Geometry: final body of the model. Coordinates: model frame, mm. Face numbers are marked on the shaded views. Give positions to 0.01 mm unless a question says otherwise; leave off trailing zeros. Order: outer loops, then holes, each group sorted by start corner. A loop starts at its lowest first (then second) coordinate and runs counter-clockwise, first axis right, second up. Notation, with made-up numbers: (-23, 7) - (-11, 7) arc R29 cw to (-11, 32) - close; hole circle Ø1 at (10.25, 7). An arc over 180 degrees is marked (long way). Use one line per item in the form item = value.
from build123d import *

# Parameters (mm, degrees)
BOSS_EXTRUDE2_DEPTH = 2.5
BOSS_EXTRUDE3_DEPTH = 5
BOSS_EXTRUDE4_START = 5
BOSS_EXTRUDE4_DEPTH = 5
SKETCH4_R           = 2.75
CUT_EXTRUDE1_DEPTH  = 10


with BuildPart() as part:
    # Sketch1 → Boss-Extrude2 (new body)
    with BuildSketch(Plane.XY):
        with BuildLine():
            ThreePointArc((-26, 0), (0, -26), (26, 0))
            Line((26, 0), (31, 0))
            Line((31, 0), (31, -41))
            Line((31, -41), (-31, -41))
            Line((-31, -41), (-31, 0))
            Line((-31, 0), (-26, 0))
        make_face()
    extrude(amount=BOSS_EXTRUDE2_DEPTH)

    # Sketch2 → Boss-Extrude3 (add)
    with BuildSketch(Plane.XY.offset(2.5)):
        with BuildLine():
            Line((-24, 0), (-31, 0))
            Line((-31, 0), (-31, -41))
            Line((-31, -41), (31, -41))
            Line((31, -41), (31, 0))
            Line((31, 0), (24, 0))
            ThreePointArc((24, 0), (0, -24), (-24, 0))
        make_face()
    extrude(amount=BOSS_EXTRUDE3_DEPTH)

    # Sketch3 → Boss-Extrude4 (add)
    with BuildSketch(Plane(origin=(0, 0, 0), x_dir=(-1, 0, 0), z_dir=(0, 0, -1)).offset(BOSS_EXTRUDE4_START)):
        with BuildLine():
            Line((-24, 0), (-31, 0))
            Line((-31, 0), (-31, -41))
            Line((-31, -41), (31, -41))
            Line((31, -41), (31, 0))
            Line((31, 0), (24, 0))
            ThreePointArc((24, 0), (0, -24), (-24, 0))
        make_face()
    extrude(amount=-BOSS_EXTRUDE4_DEPTH)

    # Sketch4 → Cut-Extrude1 (cut)
    with BuildSketch(Plane(origin=(0, -41, 0), x_dir=(-1, 0, 0), z_dir=(0, -1, 0))):
        with Locations(Location((0, -1.25, 0), (0, 0, 90))):
            Circle(SKETCH4_R)
    extrude(amount=-CUT_EXTRUDE1_DEPTH, mode=Mode.SUBTRACT)


solid = part.part
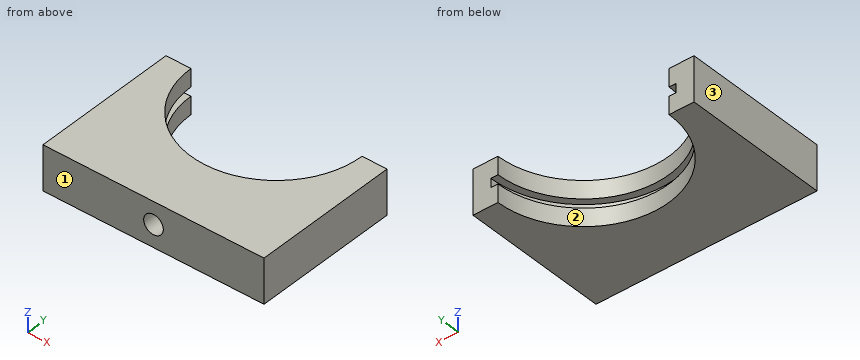
(1) Cut plane B-B on z = 1.25. Output: boundary loops of the cut face in (x, y).
Computed values:
outline = (-31, -41) - (-2.75, -41) - (-2.75, -31) - (2.75, -31) - (2.75, -41) - (31, -41) - (31, 0) - (26, 0) arc R26 cw to (-26, 0) - (-31, 0) - close
(2) Cut plane A-A on y = -37. Output: boundary loops of the cut face in (x, z), plus the area to 3 significant figures.
Computed values:
outline = (-31, -5) - (31, -5) - (31, 7.5) - (-31, 7.5) - close; hole circle Ø5.5 at (0, 1.25)
area = 751 mm²
(3) Cut plane D-D on y = -6.5. Output: boundary loops of the cut face in (x, z).
Computed values:
outline = (-31, -5) - (-23.1, -5) - (-23.1, 0) - (-25.17, 0) - (-25.17, 2.5) - (-23.1, 2.5) - (-23.1, 7.5) - (-31, 7.5) - close; (23.1, -5) - (31, -5) - (31, 7.5) - (23.1, 7.5) - (23.1, 2.5) - (25.17, 2.5) - (25.17, 0) - (23.1, 0) - close
(4) Ray query, line 1 along Z through (x, y) = (-17, -19); line 2 along X through (y, z) = (-34.75, 1.25); line 3 along X through (y, z) = (-9.5, 5.5). Return the intervals inside material, ascending.
Computed values:
line_1 = -5 to 0, 2.5 to 7.5
line_2 = -31 to -2.75, 2.75 to 31
line_3 = -31 to -22.04, 22.04 to 31
(5) Contact query for flat-ended pins moving along their axis: pin 1 Ø3.5 at (x, z) = (0, 1.25) entering from -Y; pin 2 Ø1 at (x, z) = (-9, -1) entering from +Y. Output: stop coordinate, or through.
Computed values:
pin_1 = -31
pin_2 = -22.04
(6) Pull-direction query (X, two-part tool) for the marked faces 1, 2 and 3; classes: released by +X, released by -X, zero draft, split by the parting line, or undercut.
Computed values:
face_1 = zero draft
face_2 = undercut
face_3 = released by -X
(7) Cut plane C-C on x = 0. Output: boundary loops of the cut face in (y, z), plus the area to 4 significant figures.
Computed values:
outline = (-41, -5) - (-24, -5) - (-24, 0) - (-26, 0) - (-26, 2.5) - (-24, 2.5) - (-24, 7.5) - (-41, 7.5) - (-41, 4) - (-31, 4) - (-31, -1.5) - (-41, -1.5) - close
area = 152.5 mm²
